Here's the drawing with two shaded views (mm, measured from the low corner). I have some questions. A direction names the side the tool comes from. Give positions to 0.01 mm unless a question says otherwise; leave off trailing zeros. Write each loop counter-clockwise with the first axis right and the second up, starting at its lowest first coordinate (ties: lowest second). Pieces come first, ordered by that corner, then holes.
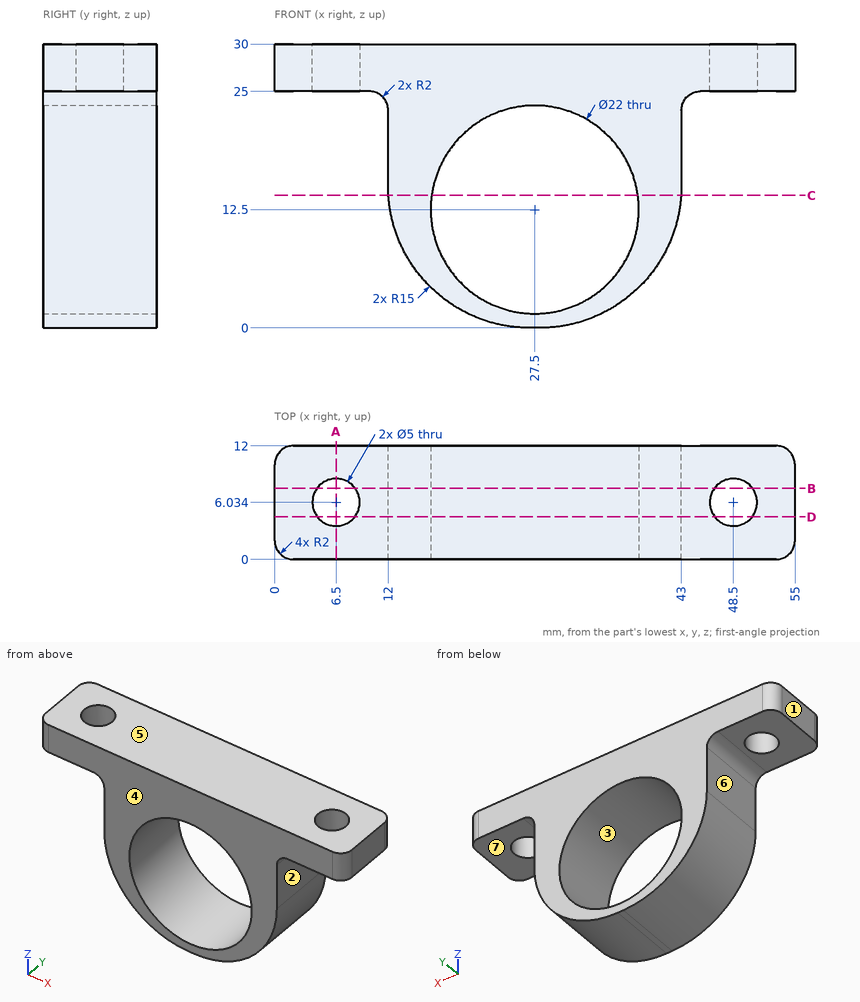
(1) For the marked faces 5, 6 and 7, which set-ups out of +Z, -Z, +X, -X, +Y, -Y let a thin tool reach every point of the face, with its end or its side?
Returned:
face 5: +Z, +X, -X, +Y, -Y
face 6: -Z, -X, +Y, -Y
face 7: -Z, +X, +Y, -Y
(2) Imagine slicing it at A-A, the plane x = 6.5. Write out the boundary of the cut face in (y, z).
Returned:
outline: (0, 25) - (3.53, 25) - (3.53, 30) - (0, 30) - close; (8.53, 25) - (12, 25) - (12, 30) - (8.53, 30) - close
(3) Imagine slicing it at D-D, the plane y = 4.5. Write out the boundary of the cut face in (x, z).
Returned:
outline: (0, 25) - (4.53, 25) - (4.53, 30) - (0, 30) - close; (8.47, 25) - (10, 25) arc R2 cw to (12, 23) - (12, 15) arc R15 ccw to (27, 0) - (28, 0) arc R15 ccw to (43, 15) - (43, 23) arc R2 cw to (45, 25) - (46.53, 25) - (46.53, 30) - (8.47, 30) - close; (50.47, 25) - (55, 25) - (55, 30) - (50.47, 30) - close; hole circle Ø22 at (27.5, 12.5)
(4) If we mould it in two halves opening along X, with no side actions, what happens to the marked faces 1, 2, 3 and 4? For each: +X half, -X half, draft (parallel to the pull), parting line (faces both ways), or undercut.
Returned:
face 1: -X half
face 2: +X half
face 3: undercut
face 4: draft
(5) Imagine slicing it at B-B, the plane y = 7.5. Write out the boundary of the cut face in (x, z) (3 decimals).
Returned:
outline: (0, 25) - (4.475, 25) - (4.475, 30) - (0, 30) - close; (8.525, 25) - (10, 25) arc R2 cw to (12, 23) - (12, 15) arc R15 ccw to (27, 0) - (28, 0) arc R15 ccw to (43, 15) - (43, 23) arc R2 cw to (45, 25) - (46.475, 25) - (46.475, 30) - (8.525, 30) - close; (50.525, 25) - (55, 25) - (55, 30) - (50.525, 30) - close; hole circle Ø22 at (27.5, 12.5)
(6) Imagine slicing it at C-C, the plane z = 14. Write out the boundary of the cut face in (x, y), plus the area to 3 significant figures.
Returned:
outline: (12.03, 0) - (16.6, 0) - (16.6, 12) - (12.03, 12) - close; (38.4, 0) - (42.97, 0) - (42.97, 12) - (38.4, 12) - close
area: 110 mm2
(7) Will these pins go through, and if not, where does the flat tip stop? P1, Ø3, axis at x = 20, z = 17.5, coming from the +Y side; P2, Ø2.5, axis at y = 8.5, z = 20, coming from the +X side; P3, Ø6, axis at x = 6.5, y = 6.03, coming from the +Z side; P4, Ø2.5, axis at y = 9, z = 20, coming from the -X side.
Returned:
P1: passes through
P2: stops at x = 43
P3: stops at z = 30
P4: stops at x = 12
(8) If I drill on L1, parallel to X at y = 7.5, z = 26 (1 decimal); L2, parallel to Y at x = 6.5, z = 28.8; L3, parallel to X at y = 4.25, z = 26, over which ranges is the centre line in solid material (lowest first)?
Returned:
L1: x = 0 to 4.5, 8.5 to 46.5, 50.5 to 55
L2: y = 0 to 3.53, 8.53 to 12
L3: x = 0 to 4.75, 8.25 to 46.75, 50.25 to 55
